Check sheet for the modelled part. Datum: model origin and axes. Units: mm. Face numbers are marked on the shaded views. A direction names the side the tool comes from. Round coordinates to 2 decimals unless told otherwise and drop trailing zeros. Write each loop counter-clockwise with the first axis right and the second up, starting at its lowest first coordinate (ties: lowest second). Pieces come first, ordered by that corner, then holes.
Item 1: Release check for a two-part mould opening along Z. For the marked faces 1, 2 and 3 record: pulls with the +Z half, pulls with the -Z half, needs draft (parallel to the pull), parting line crosses it, or undercut.
Item 2: Section check C-C, the plane y = 1.95. Record the cut outline in (x, z) (1 decimal).
Item 3: Section check A-A, the plane y = 1.2. Record the cut outline in (x, z) (1 decimal).
Item 4: Material ranges on line 1 along Y through (x, z) = (2.9, -6); line 2 along Y through (x, z) = (3.05, -1); line 3 along Y through (x, z) = (2.6, -6.25), recorded low to high.
Item 5: Depth check by flat-ended pin: pin 1 (1 mm diameter, centred on y = 4.5, z = -6.5, fed in from +X) (3 decimals); pin 2 (1.1 mm diameter, centred on y = 3, z = -0.5, fed in from +X); pin 3 (1.1 mm diameter, centred on x = 3.5, z = -5.5, fed in from +Y). Enter the tip coordinate at first touch or a pass-through.
Item 6: Set-up check for the marked faces 4, 5 and 6: record each of +Z, -Z, +X, -X, +Y, -Y from which the full face is reachable in a straight line by a thin tool's end or side.
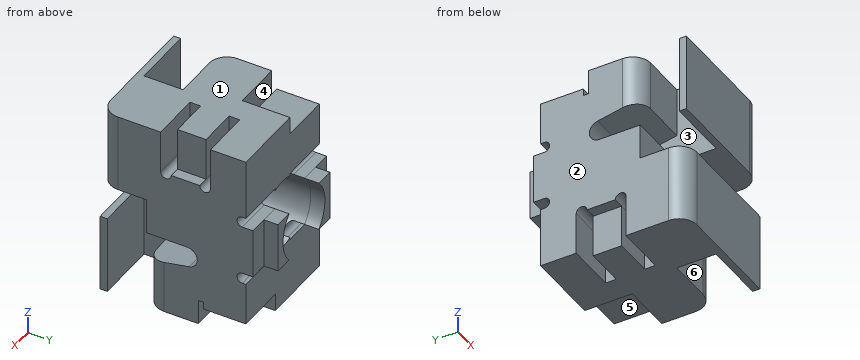
from build123d import *

# Parameters (mm, degrees)
SKETCH1_W           = 4.445
SKETCH1_H           = 6.858
BOSS_EXTRUDE1_DEPTH = 5.461
SKETCH2_R           = 1.27
CUT_EXTRUDE1_DEPTH  = 1.778
SKETCH3_W           = 1.27
SKETCH3_H           = 3.302
CUT_EXTRUDE2_DEPTH  = 10.829176466
CUT_EXTRUDE3_DEPTH  = 2.2225
CUT_EXTRUDE4_DEPTH  = 2.2225
CUT_EXTRUDE6_DEPTH  = 1.778
CUT_EXTRUDE7_START  = -1.778
CUT_EXTRUDE7_DEPTH  = 1.778
FILLET1_R           = 0.635
SKETCH14_W          = 0.889
SKETCH14_H          = 0.254
CUT_EXTRUDE8_DEPTH  = 10.829176567
BOSS_EXTRUDE2_START = 0.508
BOSS_EXTRUDE2_DEPTH = 0.508
SKETCH16_W          = 1.524
SKETCH16_H          = 1.016
CUT_EXTRUDE9_DEPTH  = 0.381
SKETCH17_W          = 1.524
SKETCH17_H          = 1.016
CUT_EXTRUDE10_DEPTH = 0.381


with BuildPart() as part:
    # Sketch1 → Boss-Extrude1 (new body)
    with BuildSketch(Plane(origin=(0, 0, 0), x_dir=(1, 0, 0), z_dir=(0, 1, 0))):
        with Locations((2.2225, 3.429)):
            Rectangle(SKETCH1_W, SKETCH1_H)
    extrude(amount=BOSS_EXTRUDE1_DEPTH)

    # Sketch2 → Cut-Extrude1 (cut)
    with BuildSketch(Plane(origin=(0, 5.461, 0), x_dir=(1, 0, 0), z_dir=(0, 1, 0))):
        with Locations(Location((2.2225, 3.429, 0), (0, 0, 270))):
            Circle(SKETCH2_R)
    extrude(amount=-CUT_EXTRUDE1_DEPTH, mode=Mode.SUBTRACT)

    # Sketch3 → Cut-Extrude2 (cut, through all)
    with BuildSketch(Plane.ZY):
        with Locations((-3.429, 0)):
            Rectangle(SKETCH3_W, SKETCH3_H)
    extrude(amount=-CUT_EXTRUDE2_DEPTH, mode=Mode.SUBTRACT)

    # Sketch4 → Cut-Extrude3 (cut)
    with BuildSketch(Plane.ZY):
        with BuildLine():
            Line((-2.794, 1.651), (-2.794, 3.11311482))
            ThreePointArc((-2.794, 3.11311482), (-2.452929401, 3.467407127), (-2.061869299, 3.169205537))
            Line((-2.061869299, 3.169205537), (-1.767735227, 1.651))
            Line((-1.767735227, 1.651), (0, 1.651))
            Line((0, 1.651), (0, 0.254))
            Line((0, 0.254), (-2.794, 0.254))
            Line((-2.794, 0.254), (-2.794, 1.651))
        make_face()
    extrude(amount=-CUT_EXTRUDE3_DEPTH, mode=Mode.SUBTRACT)

    # Sketch11 → Cut-Extrude4 (cut)
    with BuildSketch(Plane(origin=(4.445, 0, 0), x_dir=(0, 0, -1), z_dir=(1, 0, 0))):
        with BuildLine():
            Line((6.858, 0.254), (6.858, 1.651))
            Line((6.858, 1.651), (5.090264773, 1.651))
            Line((5.090264773, 1.651), (4.796130701, 3.169205537))
            ThreePointArc((4.796130701, 3.169205537), (4.405070599, 3.467407127), (4.064, 3.11311482))
            Line((4.064, 3.11311482), (4.064, 1.651))
            Line((4.064, 1.651), (4.064, 0.254))
            Line((4.064, 0.254), (6.858, 0.254))
        make_face()
    extrude(amount=-CUT_EXTRUDE4_DEPTH, mode=Mode.SUBTRACT)

    # Sketch12 → Cut-Extrude6 (cut)
    with BuildSketch(Plane(origin=(4.445, 0, 0), x_dir=(0, 0, -1), z_dir=(1, 0, 0))):
        with BuildLine():
            Line((0, 2.159), (1.524, 2.159))
            ThreePointArc((1.524, 2.159), (1.7145, 2.3495), (1.524, 2.54))
            Line((1.524, 2.54), (0, 2.54))
            Line((0, 2.54), (0, 2.159))
        make_face()
        with BuildLine():
            Line((0, 3.937), (1.524, 3.937))
            ThreePointArc((1.524, 3.937), (1.7145, 3.7465), (1.524, 3.556))
            Line((1.524, 3.556), (0, 3.556))
            Line((0, 3.556), (0, 3.937))
        make_face()
        with BuildLine():
            Line((2.54, 5.207), (2.54, 5.08))
            ThreePointArc((2.54, 5.08), (2.3495, 4.8895), (2.159, 5.08))
            Line((2.159, 5.08), (2.159, 5.207))
            Line((2.159, 5.207), (0, 5.207))
            Line((0, 5.207), (0, 5.461))
            Line((0, 5.461), (2.54, 5.461))
            Line((2.54, 5.461), (2.54, 5.207))
        make_face()
        with BuildLine():
            Line((4.699, 5.08), (4.699, 5.207))
            Line((4.699, 5.207), (6.223, 5.207))
            Line((6.223, 5.207), (6.223, 3.683))
            Line((6.223, 3.683), (5.969, 3.683))
            Line((5.969, 3.683), (5.969, 3.5052))
            Line((5.969, 3.5052), (6.858, 3.5052))
            Line((6.858, 3.5052), (6.858, 5.461))
            Line((6.858, 5.461), (4.318, 5.461))
            Line((4.318, 5.461), (4.318, 5.207))
            Line((4.318, 5.207), (4.318, 5.08))
            ThreePointArc((4.318, 5.08), (4.5085, 4.8895), (4.699, 5.08))
        make_face()
    extrude(amount=-CUT_EXTRUDE6_DEPTH, mode=Mode.SUBTRACT)

    # Sketch13 → Cut-Extrude7 (cut)
    with BuildSketch(Plane.ZY.offset(CUT_EXTRUDE7_START)):
        with BuildLine():
            Line((-6.858, 2.159), (-5.334, 2.159))
            ThreePointArc((-5.334, 2.159), (-5.1435, 2.3495), (-5.334, 2.54))
            Line((-5.334, 2.54), (-6.858, 2.54))
            Line((-6.858, 2.54), (-6.858, 2.159))
        make_face()
        with BuildLine():
            Line((-6.858, 3.937), (-5.334, 3.937))
            ThreePointArc((-5.334, 3.937), (-5.1435, 3.7465), (-5.334, 3.556))
            Line((-5.334, 3.556), (-6.858, 3.556))
            Line((-6.858, 3.556), (-6.858, 3.937))
        make_face()
        with BuildLine():
            Line((-4.318, 5.207), (-4.318, 5.08))
            ThreePointArc((-4.318, 5.08), (-4.5085, 4.8895), (-4.699, 5.08))
            Line((-4.699, 5.08), (-4.699, 5.207))
            Line((-4.699, 5.207), (-6.858, 5.207))
            Line((-6.858, 5.207), (-6.858, 5.461))
            Line((-6.858, 5.461), (-4.318, 5.461))
            Line((-4.318, 5.461), (-4.318, 5.207))
        make_face()
        with BuildLine():
            Line((-2.159, 5.08), (-2.159, 5.207))
            Line((-2.159, 5.207), (-0.635, 5.207))
            Line((-0.635, 5.207), (-0.635, 3.683))
            Line((-0.635, 3.683), (-0.889, 3.683))
            Line((-0.889, 3.683), (-0.889, 3.5052))
            Line((-0.889, 3.5052), (0, 3.5052))
            Line((0, 3.5052), (0, 5.461))
            Line((0, 5.461), (-2.54, 5.461))
            Line((-2.54, 5.461), (-2.54, 5.207))
            Line((-2.54, 5.207), (-2.54, 5.08))
            ThreePointArc((-2.54, 5.08), (-2.3495, 4.8895), (-2.159, 5.08))
        make_face()
    extrude(amount=CUT_EXTRUDE7_DEPTH, mode=Mode.SUBTRACT)

    # Fillet1
    fillet1_edges = [part.edges().sort_by_distance(p)[0] for p in [
        (0, 1.651, -0.883867613),
        (4.445, 0, -1.397),
        (0, 0, -5.461),
        (4.445, 1.651, -5.974132387),
    ]]
    fillet(fillet1_edges, radius=FILLET1_R)

    # Sketch14 → Cut-Extrude8 (cut, through all)
    with BuildSketch(Plane(origin=(0, 0, -6.858), x_dir=(-1, 0, 0), z_dir=(0, 0, -1))):
        with Locations((-2.2225, 5.334)):
            Rectangle(SKETCH14_W, SKETCH14_H)
    extrude(amount=-CUT_EXTRUDE8_DEPTH, mode=Mode.SUBTRACT)

    # Sketch15 → Boss-Extrude2 (add)
    with BuildSketch(Plane(origin=(0, 5.461, 0), x_dir=(1, 0, 0), z_dir=(0, 1, 0)).offset(BOSS_EXTRUDE2_START)):
        with BuildLine():
            Line((3.12946141, 4.318), (3.787230705, 4.318))
            Line((3.787230705, 4.318), (3.787230705, 2.54))
            Line((3.787230705, 2.54), (3.12946141, 2.54))
            ThreePointArc((3.12946141, 2.54), (3.4925, 3.429), (3.12946141, 4.318))
        make_face()
        with BuildLine():
            Line((1.31553859, 4.318), (0.657769295, 4.318))
            Line((0.657769295, 4.318), (0.657769295, 2.54))
            Line((0.657769295, 2.54), (1.31553859, 2.54))
            ThreePointArc((1.31553859, 2.54), (0.9525, 3.429), (1.31553859, 4.318))
        make_face()
    extrude(amount=-BOSS_EXTRUDE2_DEPTH)

    # Sketch16 → Cut-Extrude9 (cut)
    with BuildSketch(Plane.ZY):
        with Locations((-6.096, 3.048)):
            Rectangle(SKETCH16_W, SKETCH16_H)
    extrude(amount=-CUT_EXTRUDE9_DEPTH, mode=Mode.SUBTRACT)

    # Sketch17 → Cut-Extrude10 (cut)
    with BuildSketch(Plane(origin=(4.445, 0, 0), x_dir=(0, 0, -1), z_dir=(1, 0, 0))):
        with Locations((0.762, 3.048)):
            Rectangle(SKETCH17_W, SKETCH17_H)
    extrude(amount=-CUT_EXTRUDE10_DEPTH, mode=Mode.SUBTRACT)


solid = part.part
Values found:
1. face 1: pulls with the +Z half
1. face 2: needs draft
1. face 3: undercut
2. outline: (0, -6.9) - (4.3, -6.9) - (4.3, -5) - (2.2, -5) - (2.2, -4.1) - (4.4, -4.1) - (4.4, 0) - (0.1, 0) - (0.1, -1.8) - (2.2, -1.8) - (2.2, -2.8) - (0, -2.8) - close
3. outline: (0, -6.9) - (2.2, -6.9) - (2.2, -4.1) - (0, -4.1) - close; (2.2, -2.8) - (4.4, -2.8) - (4.4, 0) - (2.2, 0) - close
4. line 1: y = 0 to 0.25, 1.65 to 3.51, 3.68 to 5.21
4. line 2: y = 0 to 2.16, 2.54 to 3.56, 3.94 to 5.21
4. line 3: y = 0 to 0.25, 1.65 to 5.21
5. pin 1: stops at x = 4.445
5. pin 2: stops at x = 4.06
5. pin 3: stops at y = 5.21
6. face 4: +Z, -X
6. face 5: -Z, +X, +Y
6. face 6: -Z, +X
